Source: CAD feature listing. Evaluate the final solid. Frame: model axes, mm. Round coordinates to 2 decimals unless told otherwise and drop trailing zeros. Loops run counter-clockwise (first coordinate to the right, second up) from the corner with the lowest first, then second, coordinate; pieces in that order, holes last. Notation, with made-up numbers: (4, -13) - (39, -13) arc R23 ccw to (39, 4) - close; hole circle Ø3 at (70, -5). An arc over 180 degrees is marked (long way). One line per question, with ' | ' between items.
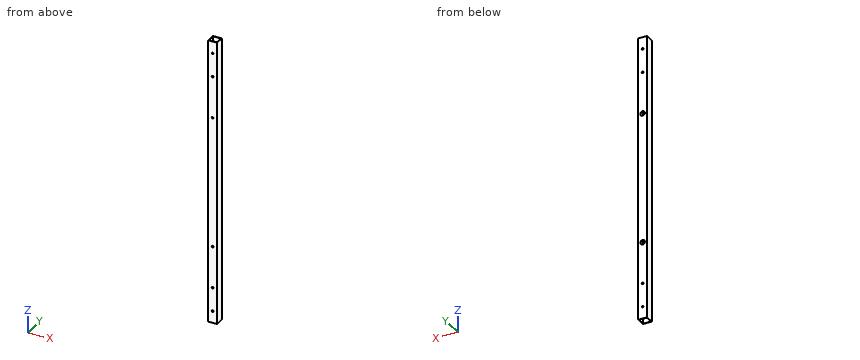
from build123d import *

# Parameters (mm, degrees)
SKETCH_1_W          = 15
SKETCH_1_H          = 15
SKETCH_1_W_2        = 13
SKETCH_1_H_2        = 13
EXTRUDE_1_DEPTH     = 460
SKETCH_2_R          = 1.5
CUT_EXTRUDE_1_DEPTH = 480
SKETCH_3_R          = 4
CUT_EXTRUDE_2_DEPTH = 2
SKETCH_4_W          = 15
SKETCH_4_H          = 15
EXTRUDE_2_DEPTH     = 10
SKETCH_5_W          = 15
SKETCH_5_H          = 15
EXTRUDE_3_DEPTH     = 10
SKETCH_6_W          = 13
SKETCH_6_H          = 13
CUT_EXTRUDE_3_DEPTH = 481.117173198
SKETCH_7_R          = 1.5
CUT_EXTRUDE_4_DEPTH = 471.299106952


with BuildPart() as part:
    # 草图1 → 凸台-拉伸1 (new body)
    with BuildSketch(Plane.XY):
        Rectangle(SKETCH_1_W, SKETCH_1_H)
        Rectangle(SKETCH_1_W_2, SKETCH_1_H_2, mode=Mode.SUBTRACT)
    extrude(amount=EXTRUDE_1_DEPTH)

    # 草图2 → 切除-拉伸1 (cut)
    with BuildSketch(Plane(origin=(0, 7.5, 0), x_dir=(1, 0, 0), z_dir=(0, 1, 0))):
        with Locations(Location((0, -120, 0), (0, 0, 270))):
            Circle(SKETCH_2_R)
        with Locations((0, -340)):
            Circle(SKETCH_2_R)
    extrude(amount=-CUT_EXTRUDE_1_DEPTH, mode=Mode.SUBTRACT)

    # 草图3 → 切除-拉伸2 (cut)
    with BuildSketch(Plane(origin=(0, 7.5, 0), x_dir=(1, 0, 0), z_dir=(0, 1, 0))):
        with Locations(Location((0, -120, 0), (0, 0, 270))):
            Circle(SKETCH_3_R)
        with Locations(Location((0, -340, 0), (0, 0, 270))):
            Circle(SKETCH_3_R)
    extrude(amount=-CUT_EXTRUDE_2_DEPTH, mode=Mode.SUBTRACT)

    # 草图4 → 凸台-拉伸2 (add)
    with BuildSketch(Plane(origin=(0, 0, 0), x_dir=(-1, 0, 0), z_dir=(0, 0, -1))):
        Rectangle(SKETCH_4_W, SKETCH_4_H)
    extrude(amount=EXTRUDE_2_DEPTH)

    # 草图5 → 凸台-拉伸3 (add)
    with BuildSketch(Plane.XY.offset(460)):
        Rectangle(SKETCH_5_W, SKETCH_5_H)
    extrude(amount=EXTRUDE_3_DEPTH)

    # 草图6 → 切除-拉伸3 (cut, through all)
    with BuildSketch(Plane.XY.offset(470)):
        Rectangle(SKETCH_6_W, SKETCH_6_H)
    extrude(amount=-CUT_EXTRUDE_3_DEPTH, mode=Mode.SUBTRACT)

    # 草图7 → 切除-拉伸4 (cut, through all)
    with BuildSketch(Plane.XZ.offset(7.5)):
        with Locations(Location((0, 10, 0), (0, 0, 270))):
            Circle(SKETCH_7_R)
        with Locations(Location((0, 50, 0), (0, 0, 270))):
            Circle(SKETCH_7_R)
        with Locations((0, 450)):
            Circle(SKETCH_7_R)
        with Locations((0, 410)):
            Circle(SKETCH_7_R)
    extrude(amount=-CUT_EXTRUDE_4_DEPTH, mode=Mode.SUBTRACT)


solid = part.part
1. Contact query for flat-ended pins moving along their axis: P1, Ø1.8, axis at x = 0, z = 10, coming from the -Y side; P2, Ø6.5, axis at x = 0, z = 340, coming from the +Y side. Output: stop coordinate, or through.
Worked out:
P1: passes through | P2: stops at y = -6.5
2. Material intervals for probe 1 along Y at (x, z) = (2.25, 132); probe 2 along X at (y, z) = (6.9, 10), sorted ascending.
Worked out:
probe 1: y = -7.5 to -6.5, 6.5 to 7.5 | probe 2: x = -7.5 to -1.5, 1.5 to 7.5
3. Section query B-B, the plane z = 96. Return loops of the section in (x, y), plus the area to 3 significant figures.
Worked out:
outline: (-7.5, -7.5) - (7.5, -7.5) - (7.5, 7.5) - (-7.5, 7.5) - close; hole (-6.5, -6.5) - (6.5, -6.5) - (6.5, 6.5) - (-6.5, 6.5) - close | area: 56.0 mm2
4. Section query A-A, the plane y = 1.5. Return loops of the section in (x, z).
Worked out:
outline: (-7.5, -10) - (-6.5, -10) - (-6.5, 470) - (-7.5, 470) - close; (6.5, -10) - (7.5, -10) - (7.5, 470) - (6.5, 470) - close
